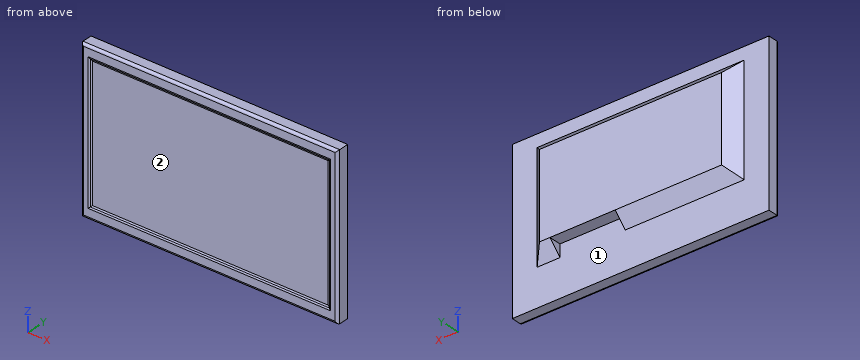
from build123d import *

# Parameters (mm, degrees)
F0_W         = 525.1352317132
F0_H         = 324.7600756863
F0_W_2       = 487.0352317132
F0_H_2       = 273.9600756863
F1_DEPTH     = 25.4
F2_DEPTH     = 22.86
F3_T1_DEPTH  = 550.5352317132
F3_T3_DEPTH  = 350.1600756863
F3_T5_DEPTH  = 487.0352317132
F3_T7_DEPTH  = 273.9600756863
F3_T13_DEPTH = 498.0337543413
F3_T17_DEPTH = 284.9585983143
F3_T24_DEPTH = 498.0337543413
F3_T28_DEPTH = 284.9585983143
F3_T35_DEPTH = 284.9585983143
F3_T39_DEPTH = 498.0337543413
F3_T46_DEPTH = 498.0337543413
F3_T50_DEPTH = 284.9585983143
F4_R         = 5.08
F5_W         = 423.5352317132
F5_H         = 223.1600756863
F6_DEPTH     = 25.4
F6_TAPER     = 45
F7_W         = 133.505359292
F7_H         = 25.4
F8_DEPTH     = 25.4


# Not quite as in the source:
# - a fillet or chamfer that OpenCascade refuses, or shapes differently, is made with other operations: its cross-section is extruded or revolved along the edge and cut away or added


with BuildPart() as f1:
    # F0 (on Front) → F1 (new body)
    with BuildSketch(Plane.XZ):
        Rectangle(F0_W, F0_H)
        Rectangle(F0_W_2, F0_H_2, mode=Mode.SUBTRACT)
    extrude(amount=F1_DEPTH)

    # F0 (on Front) → F2 (join)
    with BuildSketch(Plane.XZ):
        Polygon((-243.5176158566, 136.9800378431), (-243.5176158566, -136.9800378431), (243.5176158566, 136.9800378431), align=None)
        Polygon((-243.5176158566, -136.9800378431), (243.5176158566, -136.9800378431), (243.5176158566, 136.9800378431), align=None)
    extrude(amount=F2_DEPTH)

    # F3: fillet of radius 5.08 on 8 edges, made by hand

    # F3_s2 → F3_t1 (cut)
    with BuildSketch(Plane.YZ.offset(-275.2676158566)):
        with BuildLine():
            ThreePointArc((-20.32, 162.3800378431), (-23.9121024484, 160.8921402916), (-25.4, 157.3000378431))
            Line((-25.4, 157.3000378431), (-25.4, 162.3800378431))
            Line((-25.4, 162.3800378431), (-20.32, 162.3800378431))
        make_face()
        with BuildLine():
            ThreePointArc((-25.4, -157.3000378431), (-23.9121024484, -160.8921402916), (-20.32, -162.3800378431))
            Line((-20.32, -162.3800378431), (-25.4, -162.3800378431))
            Line((-25.4, -162.3800378431), (-25.4, -157.3000378431))
        make_face()
    extrude(amount=F3_T1_DEPTH, mode=Mode.SUBTRACT)

    # F3_s4 → F3_t3 (cut)
    with BuildSketch(Plane.XY.offset(-175.0800378431)):
        with BuildLine():
            ThreePointArc((-262.5676158566, -20.32), (-261.079718305, -23.9121024484), (-257.4876158566, -25.4))
            Line((-257.4876158566, -25.4), (-262.5676158566, -25.4))
            Line((-262.5676158566, -25.4), (-262.5676158566, -20.32))
        make_face()
        with BuildLine():
            ThreePointArc((262.5676158566, -20.32), (261.079718305, -23.9121024484), (257.4876158566, -25.4))
            Line((257.4876158566, -25.4), (262.5676158566, -25.4))
            Line((262.5676158566, -25.4), (262.5676158566, -20.32))
        make_face()
    extrude(amount=F3_T3_DEPTH, mode=Mode.SUBTRACT)

    # F3_s6 → F3_t5 (cut)
    with BuildSketch(Plane.YZ.offset(-243.5176158566)):
        with BuildLine():
            ThreePointArc((-25.4, 141.3794468944), (-24.7194090512, 138.8394468944), (-22.86, 136.9800378431))
            Line((-22.86, 136.9800378431), (-25.4, 136.9800378431))
            Line((-25.4, 136.9800378431), (-25.4, 141.3794468944))
        make_face()
        with BuildLine():
            ThreePointArc((-25.4, -141.3794468944), (-24.7194090512, -138.8394468944), (-22.86, -136.9800378431))
            Line((-22.86, -136.9800378431), (-25.4, -136.9800378431))
            Line((-25.4, -136.9800378431), (-25.4, -141.3794468944))
        make_face()
    extrude(amount=F3_T5_DEPTH, mode=Mode.SUBTRACT)

    # F3_s8 → F3_t7 (cut)
    with BuildSketch(Plane.XY.offset(-136.9800378431)):
        with BuildLine():
            ThreePointArc((247.9170249078, -25.4), (245.3770249078, -24.7194090512), (243.5176158566, -22.86))
            Line((243.5176158566, -22.86), (243.5176158566, -25.4))
            Line((243.5176158566, -25.4), (247.9170249078, -25.4))
        make_face()
        with BuildLine():
            ThreePointArc((-247.9170249078, -25.4), (-245.3770249078, -24.7194090512), (-243.5176158566, -22.86))
            Line((-243.5176158566, -22.86), (-243.5176158566, -25.4))
            Line((-243.5176158566, -25.4), (-247.9170249078, -25.4))
        make_face()
    extrude(amount=F3_T7_DEPTH, mode=Mode.SUBTRACT)


with BuildPart() as f3_tool11:
    # F3_s12 → F3_t13 (new body)
    with BuildSketch(Plane.YZ.offset(-254.5161384847)):
        with BuildLine():
            ThreePointArc((-25.4, 141.3794468944), (-24.7194090512, 138.8394468944), (-22.86, 136.9800378431))
            Line((-22.86, 136.9800378431), (-25.4, 136.9800378431))
            Line((-25.4, 136.9800378431), (-25.4, 141.3794468944))
        make_face()
    extrude(amount=F3_T13_DEPTH)

    split(bisect_by=Plane.YZ.offset(-243.5176158566), keep=Keep.BOTTOM)


with BuildPart() as f3_tool15:
    # F3_s16 → F3_t17 (new body)
    with BuildSketch(Plane.XY.offset(-136.9800378431)):
        with BuildLine():
            ThreePointArc((-247.9170249078, -25.4), (-245.3770249078, -24.7194090512), (-243.5176158566, -22.86))
            Line((-243.5176158566, -22.86), (-243.5176158566, -25.4))
            Line((-243.5176158566, -25.4), (-247.9170249078, -25.4))
        make_face()
    extrude(amount=F3_T17_DEPTH)

    split(bisect_by=Plane.XY.offset(136.9800378431), keep=Keep.TOP)


with BuildPart() as f3_tool11_1:
    add(f3_tool11.part)

    # F3_t19: intersect F3_tool15
    add(f3_tool15.part, mode=Mode.INTERSECT)


with BuildPart() as f1_1:
    add(f1.part)

    # F3_t9: cut F3_tool11
    add(f3_tool11_1.part, mode=Mode.SUBTRACT)


with BuildPart() as f3_tool22:
    # F3_s23 → F3_t24 (new body)
    with BuildSketch(Plane.YZ.offset(-243.5176158566)):
        with BuildLine():
            ThreePointArc((-25.4, 141.3794468944), (-24.7194090512, 138.8394468944), (-22.86, 136.9800378431))
            Line((-22.86, 136.9800378431), (-25.4, 136.9800378431))
            Line((-25.4, 136.9800378431), (-25.4, 141.3794468944))
        make_face()
    extrude(amount=F3_T24_DEPTH)

    split(bisect_by=Plane.YZ.offset(243.5176158566), keep=Keep.TOP)


with BuildPart() as f3_tool26:
    # F3_s27 → F3_t28 (new body)
    with BuildSketch(Plane.XY.offset(147.9785604712)):
        with BuildLine():
            ThreePointArc((247.9170249078, -25.4), (245.3770249078, -24.7194090512), (243.5176158566, -22.86))
            Line((243.5176158566, -22.86), (243.5176158566, -25.4))
            Line((243.5176158566, -25.4), (247.9170249078, -25.4))
        make_face()
    extrude(amount=-F3_T28_DEPTH)

    split(bisect_by=Plane.XY.offset(136.9800378431), keep=Keep.TOP)


with BuildPart() as f3_tool22_1:
    add(f3_tool22.part)

    # F3_t30: intersect F3_tool26
    add(f3_tool26.part, mode=Mode.INTERSECT)


with BuildPart() as f1_2:
    add(f1_1.part)

    # F3_t20: cut F3_tool22
    add(f3_tool22_1.part, mode=Mode.SUBTRACT)


with BuildPart() as f3_tool33:
    # F3_s34 → F3_t35 (new body)
    with BuildSketch(Plane.XY.offset(136.9800378431)):
        with BuildLine():
            ThreePointArc((247.9170249078, -25.4), (245.3770249078, -24.7194090512), (243.5176158566, -22.86))
            Line((243.5176158566, -22.86), (243.5176158566, -25.4))
            Line((243.5176158566, -25.4), (247.9170249078, -25.4))
        make_face()
    extrude(amount=-F3_T35_DEPTH)

    split(bisect_by=Plane.XY.offset(-136.9800378431), keep=Keep.BOTTOM)


with BuildPart() as f3_tool37:
    # F3_s38 → F3_t39 (new body)
    with BuildSketch(Plane.YZ.offset(254.5161384847)):
        with BuildLine():
            ThreePointArc((-25.4, -141.3794468944), (-24.7194090512, -138.8394468944), (-22.86, -136.9800378431))
            Line((-22.86, -136.9800378431), (-25.4, -136.9800378431))
            Line((-25.4, -136.9800378431), (-25.4, -141.3794468944))
        make_face()
    extrude(amount=-F3_T39_DEPTH)

    split(bisect_by=Plane.YZ.offset(243.5176158566), keep=Keep.TOP)


with BuildPart() as f3_tool33_1:
    add(f3_tool33.part)

    # F3_t41: intersect F3_tool37
    add(f3_tool37.part, mode=Mode.INTERSECT)


with BuildPart() as f1_3:
    add(f1_2.part)

    # F3_t31: cut F3_tool33
    add(f3_tool33_1.part, mode=Mode.SUBTRACT)


with BuildPart() as f3_tool44:
    # F3_s45 → F3_t46 (new body)
    with BuildSketch(Plane.YZ.offset(243.5176158566)):
        with BuildLine():
            ThreePointArc((-25.4, -141.3794468944), (-24.7194090512, -138.8394468944), (-22.86, -136.9800378431))
            Line((-22.86, -136.9800378431), (-25.4, -136.9800378431))
            Line((-25.4, -136.9800378431), (-25.4, -141.3794468944))
        make_face()
    extrude(amount=-F3_T46_DEPTH)

    split(bisect_by=Plane.YZ.offset(-243.5176158566), keep=Keep.BOTTOM)


with BuildPart() as f3_tool48:
    # F3_s49 → F3_t50 (new body)
    with BuildSketch(Plane.XY.offset(-147.9785604712)):
        with BuildLine():
            ThreePointArc((-247.9170249078, -25.4), (-245.3770249078, -24.7194090512), (-243.5176158566, -22.86))
            Line((-243.5176158566, -22.86), (-243.5176158566, -25.4))
            Line((-243.5176158566, -25.4), (-247.9170249078, -25.4))
        make_face()
    extrude(amount=F3_T50_DEPTH)

    split(bisect_by=Plane.XY.offset(-136.9800378431), keep=Keep.BOTTOM)


with BuildPart() as f3_tool44_1:
    add(f3_tool44.part)

    # F3_t52: intersect F3_tool48
    add(f3_tool48.part, mode=Mode.INTERSECT)


with BuildPart() as f1_4:
    add(f1_3.part)

    # F3_t42: cut F3_tool44
    add(f3_tool44_1.part, mode=Mode.SUBTRACT)

    # F4
    f4_edges = [f1_4.edges().sort_by_distance(p)[0] for p in [
        (0, -22.86, 136.980038),
        (-243.517616, -22.86, 0),
        (0, -22.86, -136.980038),
        (243.517616, -22.86, 0),
    ]]
    fillet(f4_edges, radius=F4_R)

    # F5 (on face) → F6 (join)
    with BuildSketch(Plane(origin=(0, 0, 0), x_dir=(-1, 0, 0), z_dir=(0, 1, 0))):
        with Locations((0, 25.4)):
            Rectangle(F5_W, F5_H)
    extrude(amount=F6_DEPTH, taper=F6_TAPER)

    # F7 (on face) → F8 (cut)
    with BuildSketch(Plane(origin=(0, 0, 0), x_dir=(-1, 0, 0), z_dir=(0, 1, 0))):
        with Locations((-98.213173449, -73.4800378431)):
            Rectangle(F7_W, F7_H)
    extrude(amount=F8_DEPTH, mode=Mode.SUBTRACT)


solid = f1_4.part
Work out the finished part from the listing and answer in its coordinate system (mm). Face numbers are marked on the shaded views. Round coordinates to 2 decimals unless told otherwise and drop trailing zeros. Write each loop counter-clockwise with the first axis right and the second up, starting at its lowest first coordinate (ties: lowest second). Pieces come first, ordered by that corner, then holes. Notation, with made-up numbers: (56.5, -5) - (110.5, -5) arc R30 cw to (110.5, 26) - close; hole circle Ø5 at (30.25, 47). An arc over 180 degrees is marked (long way). Answer in a Markdown table with one row per item. Add a question column.
1. A cutting plane is placed at A-A, the plane z = -104. Determine the outline of the cut face in (x, y).
2. Find the intervals of material crossed by line 1 along Y through (x, z) = (-129, 102); line 2 along Y through (x, z) = (-165.5, -142); line 3 along Z through (x, y) = (-194, 13), in increasing order. Write a range as from..to.
3. Given pin 1 (5 mm diameter, centred on x = -179.5, z = -106, fed in from +Y); pin 2 (1.5 mm diameter, centred on x = -174, z = -79, fed in from +Y); pin 3 (12.5 mm diameter, centred on y = 7.5, z = -67.5, fed in from +X), each flat-ended and moving along its own axis, determine where each tip first touches the part or whether it passes through.
4. The mould has two halves that part along Z. Classify the marked faces 1 and 2: +Z half, -Z half, draft (parallel to the pull), parting line (faces both ways), or undercut.
Worked out:
| question | item | result |
|---|---|---|
| 1 | outline | (-262.57, -20.32) arc R5.08 ccw to (-257.49, -25.4) - (-247.92, -25.4) arc R5.08 ccw to (-244.56, -24.13) arc R5.08 cw to (-241.2, -22.86) - (241.2, -22.86) arc R5.08 cw to (244.56, -24.13) arc R5.08 ccw to (247.92, -25.4) - (257.49, -25.4) arc R5.08 ccw to (262.57, -20.32) - (262.57, 0) - (-262.57, 0) - close |
| 2 | line 1 | -22.86..25.4 |
| 2 | line 2 | -25.4..0 |
| 2 | line 3 | -73.18..123.98 |
| 3 | pin 1 | y = 0 |
| 3 | pin 2 | y = 7.93 |
| 3 | pin 3 | x = 210.52 |
| 4 | face 1 | draft |
| 4 | face 2 | undercut |
